Build history of the part. All positions in model axes, mm. A direction names the side the tool comes from. Give positions to 0.01 mm unless a question says otherwise; leave off trailing zeros. Order: outer loops, then holes, each group sorted by start corner. A loop starts at its lowest first (then second) coordinate and runs counter-clockwise, first axis right, second up. Notation, with made-up numbers: (74, -31) - (97, -31) arc R12 ccw to (97, -13) - close; hole circle Ø8 at (-33.5, -32). An arc over 180 degrees is marked (long way). Use a Markdown table: item, result. Add a question column.
(1) Slice it at B-B (x = 59). Write the cut outline in (y, z), then the cut area to 3 significant figures.
(2) Slice it at A-A (y = 12). Write the cut outline in (x, z), then the cut area to 3 significant figures.
(3) Flat gauge pins, fed straight in: pin 1 (8 mm diameter, centred on x = 115, z = -13.5, fed in from +Y); pin 2 (20 mm diameter, centred on x = -262.5, y = 12.5, fed in from -Z); pin 3 (10 mm diameter, centred on x = -217, z = 53.5, fed in from -Y). Where does each tip first touch, or does it go through?
(4) Mould opens along Z. For faces 4 (the face through (264.464, 37.468, -138.242)), 5 (the face through (274.5, 71, 1)), 6 (the face through (249, 0, -122)) say: +Z half, -Z half, draft (parallel to the pull), parting line (faces both ways), or undercut.
(5) Slice it at C-C (z = 29). Write the cut outline in (x, y).
(6) Wall check: line 1 (Y direction, x = -148, z = 21); line 2 (Z direction, x = 67, y = 71.5); line 3 (Z direction, x = -245, y = 67.5). Give the ranges that are in metal, low to high.
(7) Slice it at D-D (x = 223). Write the cut outline in (y, z), then the cut area to 3 significant figures.
(8) Which spindle directions (+Z, -Z, +X, -X, +Y, -Y) get a long thin tool onto all of the face, cutting with end or side? Do faces 1 (the face through (251.788, 31.986, -96.797)), 2 (the face through (229.5, 9, -127)), 3 (the face through (261.668, 71.07, -133.968)). Say none if no direction does.
from build123d import *

# Parameters (mm, degrees)
BOSS_EXTRUDE1_DEPTH = 76
CUT_EXTRUDE1_DEPTH  = 10
CUT_EXTRUDE2_DEPTH  = 421.62007798
CUT_EXTRUDE3_DEPTH  = 585.391350039


with BuildPart() as part:
    # Sketch1 → Boss-Extrude1 (new body)
    with BuildSketch(Plane(origin=(0, 0, 0), x_dir=(1, 0, 0), z_dir=(0, 1, 0))):
        with BuildLine():
            Line((-229.5, 152.5), (229.5, 152.5))
            ThreePointArc((229.5, 152.5), (264.855339059, 137.855339059), (279.5, 102.5))
            Line((279.5, 102.5), (279.5, -102.5))
            ThreePointArc((279.5, -102.5), (264.855339059, -137.855339059), (229.5, -152.5))
            Line((229.5, -152.5), (-229.5, -152.5))
            ThreePointArc((-229.5, -152.5), (-264.855339059, -137.855339059), (-279.5, -102.5))
            Line((-279.5, -102.5), (-279.5, 102.5))
            ThreePointArc((-279.5, 102.5), (-264.855339059, 137.855339059), (-229.5, 152.5))
        make_face()
    extrude(amount=BOSS_EXTRUDE1_DEPTH)

    # Sketch3 → Cut-Extrude1 (cut)
    with BuildSketch(Plane(origin=(0, 76, 0), x_dir=(1, 0, 0), z_dir=(0, 1, 0))):
        with BuildLine():
            Line((-274.5, 102.5), (-274.5, -102.5))
            ThreePointArc((-274.5, -102.5), (-261.319805153, -134.319805153), (-229.5, -147.5))
            Line((-229.5, -147.5), (229.5, -147.5))
            ThreePointArc((229.5, -147.5), (261.319805153, -134.319805153), (274.5, -102.5))
            Line((274.5, -102.5), (274.5, 102.5))
            ThreePointArc((274.5, 102.5), (261.319805153, 134.319805153), (229.5, 147.5))
            Line((229.5, 147.5), (-229.5, 147.5))
            ThreePointArc((-229.5, 147.5), (-261.319805153, 134.319805153), (-274.5, 102.5))
        make_face()
    extrude(amount=-CUT_EXTRUDE1_DEPTH, mode=Mode.SUBTRACT)

    # Sketch4 → Cut-Extrude2 (cut, through all)
    with BuildSketch(Plane.XY.offset(152.5)):
        with BuildLine():
            Line((-229.5, 0), (-229.5, 18))
            ThreePointArc((-229.5, 18), (-223.642135624, 32.142135624), (-209.5, 38))
            Line((-209.5, 38), (209.5, 38))
            ThreePointArc((209.5, 38), (223.642135624, 32.142135624), (229.5, 18))
            Line((229.5, 18), (229.5, 0))
            Line((229.5, 0), (-229.5, 0))
        make_face()
    extrude(amount=-CUT_EXTRUDE2_DEPTH, mode=Mode.SUBTRACT)

    # Sketch5 → Cut-Extrude3 (cut, through all)
    with BuildSketch(Plane.ZY.offset(279.5)):
        with BuildLine():
            Line((-102.5, 0), (-102.5, 18))
            ThreePointArc((-102.5, 18), (-96.642135624, 32.142135624), (-82.5, 38))
            Line((-82.5, 38), (82.5, 38))
            ThreePointArc((82.5, 38), (96.642135624, 32.142135624), (102.5, 18))
            Line((102.5, 18), (102.5, 0))
            Line((102.5, 0), (-102.5, 0))
        make_face()
    extrude(amount=-CUT_EXTRUDE3_DEPTH, mode=Mode.SUBTRACT)


solid = part.part
Solution:
| question | item | result |
|---|---|---|
| 1 | outline | (38, -152.5) - (76, -152.5) - (76, -147.5) - (66, -147.5) - (66, 147.5) - (76, 147.5) - (76, 152.5) - (38, 152.5) - close |
| 1 | area | 8,640 mm2 |
| 2 | outline | (-279.5, -102.5) arc R50 ccw to (-229.5, -152.5) - (-229.5, -102.5) - close; (-279.5, 102.5) - (-229.5, 102.5) - (-229.5, 152.5) arc R50 ccw to start; (229.5, -152.5) arc R50 ccw to (279.5, -102.5) - (229.5, -102.5) - close; (229.5, 102.5) - (279.5, 102.5) arc R50 ccw to (229.5, 152.5) - close |
| 2 | area | 7,850 mm2 |
| 3 | pin 1 | y = 66 |
| 3 | pin 2 | z = -146.9 |
| 3 | pin 3 | y = 38 |
| 4 | face 4 | -Z half |
| 4 | face 5 | undercut |
| 4 | face 6 | draft |
| 5 | outline | (-279.5, 38) - (279.5, 38) - (279.5, 76) - (274.5, 76) - (274.5, 66) - (-274.5, 66) - (-274.5, 76) - (-279.5, 76) - close |
| 6 | line 1 | 38 to 66 |
| 6 | line 2 | -152.5 to -147.5, 147.5 to 152.5 |
| 6 | line 3 | -150.04 to -144.75, 144.75 to 150.04 |
| 7 | outline | (32.76, -152.5) - (76, -152.5) - (76, -147.5) - (66, -147.5) - (66, 147.5) - (76, 147.5) - (76, 152.5) - (32.76, 152.5) - (32.76, 96) arc R20 cw to (38, 82.5) - (38, -82.5) arc R20 cw to (32.76, -96) - close |
| 7 | area | 9,280 mm2 |
| 8 | face 1 | +X, -X, -Y |
| 8 | face 2 | +Z, -Z, -Y |
| 8 | face 3 | +Y |
